Can you work these out from the model? Positions are in its coordinate system, mm. Give positions to 0.01 mm unless a question says otherwise; leave off trailing zeros. Loops run counter-clockwise (first coordinate to the right, second up) from the corner with the lowest first, then second, coordinate; pieces in that order, holes last. Notation, with made-up numbers: M 73,68 L 92,68 A11 ccw 92,81 Z; hole C 24.25,-26 d8. An arc over 180 degrees is marked long. Put each result on its own line as item: value. Start each with the question number.
1) For P1, Ø0.5, axis at y = 20.5, z = -0.5, coming from the -X side, with a flat end and sliding along its axis, tell me the tip position at first contact or that it passes through.
2) Imagine slicing it at B-B (x = 51.36). Write out the boundary of the cut face in (y, z), then the cut area to 3 significant figures.
3) Please list where these lines run through material, in increasing order: line 1 along X through (y, z) = (20.32, -0.7) (3 decimals); line 2 along X through (y, z) = (16.5, -0.75) (3 decimals); line 3 along Y through (x, z) = (48.5, -1.1). Write a range as from..to.
4) Imagine slicing it at C-C (z = -1.05). State how many separate pieces and enclosed holes the cut face has, then the cut area to 3 significant figures.
5) Imagine slicing it at A-A (y = 29.21). Write out the boundary of the cut face in (x, z) (3 decimals).
6) If we mould it in two halves opening along X, with no side actions, what happens to faces 1 (the cylindrical face through (17.4, 34.05, -0.79)), 2 (the cylindrical face through (52.055, 37.498, -0.789)), 3 (the cylindrical face through (45.35, 13.06, -0.79)), 4 (the flat face through (28, 19, -1.6))? For each: +X half, -X half, draft (parallel to the pull), parting line (faces both ways), or undercut.
from build123d import *

# Parameters (mm, degrees)
SKETCH_20_R         = 1.5
SKETCH_20_R_2       = 1.05
BOSS_EXTRUDE1_DEPTH = 1.6
SKETCH_17_R         = 0.8255
SKETCH_17_R_2       = 0.4191
SKETCH_17_R_3       = 0.41275
SKETCH_17_R_4       = 0.4699
SKETCH_17_R_5       = 0.829
CUT_EXTRUDE1_DEPTH  = 1.6


with BuildPart() as part:
    # Sketch 20 → Boss-Extrude1 (new body)
    with BuildSketch(Plane.XY):
        with BuildLine():
            Line((50.205, 38.4048), (6.31, 38.4048))
            ThreePointArc((6.31, 38.4048), (4.47911474, 37.520159965), (3.81, 35.6))
            Line((3.81, 35.6), (3.81, 2.5))
            ThreePointArc((3.81, 2.5), (4.542233047, 0.732233047), (6.31, 0))
            Line((6.31, 0), (50.205, 0))
            ThreePointArc((50.205, 0), (51.972766953, 0.732233047), (52.705, 2.5))
            Line((52.705, 2.5), (52.705, 35.6))
            ThreePointArc((52.705, 35.6), (52.03588526, 37.520159965), (50.205, 38.4048))
        make_face()
        with Locations((6.096, 2.1336)):
            Circle(SKETCH_20_R, mode=Mode.SUBTRACT)
        with Locations((50.5968, 2.1336)):
            Circle(SKETCH_20_R, mode=Mode.SUBTRACT)
        with Locations((50.5968, 36.2712)):
            Circle(SKETCH_20_R, mode=Mode.SUBTRACT)
        with Locations((6.096, 36.2712)):
            Circle(SKETCH_20_R, mode=Mode.SUBTRACT)
        with Locations((51.36, 12.26)):
            Circle(SKETCH_20_R_2, mode=Mode.SUBTRACT)
        with Locations((51.36, 20.76)):
            Circle(SKETCH_20_R_2, mode=Mode.SUBTRACT)
        with Locations((51.36, 24.96)):
            Circle(SKETCH_20_R_2, mode=Mode.SUBTRACT)
        with Locations((51.36, 33.46)):
            Circle(SKETCH_20_R_2, mode=Mode.SUBTRACT)
    extrude(amount=-BOSS_EXTRUDE1_DEPTH)

    # Sketch 17 → Cut-Extrude1 (cut)
    with BuildSketch(Plane.XY):
        with Locations((9.6012, 22.7838)):
            Circle(SKETCH_17_R)
        with Locations((12.319, 18.014)):
            Circle(SKETCH_17_R_2)
        with Locations((14.3002, 18.014)):
            Circle(SKETCH_17_R_2)
        with Locations((9.6012, 10.7442)):
            Circle(SKETCH_17_R)
        with Locations((20.066, 2.794)):
            Circle(SKETCH_17_R_3)
        with Locations((22.606, 2.794)):
            Circle(SKETCH_17_R_3)
        with Locations((25.146, 2.794)):
            Circle(SKETCH_17_R_3)
        with Locations((27.686, 2.794)):
            Circle(SKETCH_17_R_3)
        with Locations((22.606, 6.604)):
            Circle(SKETCH_17_R_3)
        with Locations((27.686, 6.604)):
            Circle(SKETCH_17_R_3)
        with Locations((17.145, 13.97)):
            Circle(SKETCH_17_R_3)
        with Locations((12.319, 15.514)):
            Circle(SKETCH_17_R_2)
        with Locations((14.3002, 15.514)):
            Circle(SKETCH_17_R_2)
        with Locations((14.605, 33.655)):
            Circle(SKETCH_17_R_4)
        with Locations((17.145, 33.655)):
            Circle(SKETCH_17_R_4)
        with Locations((19.685, 33.655)):
            Circle(SKETCH_17_R_4)
        with Locations((22.225, 33.655)):
            Circle(SKETCH_17_R_4)
        with Locations((24.765, 33.655)):
            Circle(SKETCH_17_R_4)
        with Locations((27.305, 33.655)):
            Circle(SKETCH_17_R_4)
        with Locations((29.845, 33.655)):
            Circle(SKETCH_17_R_4)
        with Locations((32.385, 33.655)):
            Circle(SKETCH_17_R_4)
        with Locations((34.925, 33.655)):
            Circle(SKETCH_17_R_4)
        with Locations((37.465, 33.655)):
            Circle(SKETCH_17_R_4)
        with Locations((40.005, 33.655)):
            Circle(SKETCH_17_R_4)
        with Locations((44.56, 32.91)):
            Circle(SKETCH_17_R_5)
        with Locations((48.26, 29.21)):
            Circle(SKETCH_17_R_5)
        with Locations((44.56, 25.51)):
            Circle(SKETCH_17_R_5)
        with Locations((44.56, 20.21)):
            Circle(SKETCH_17_R_5)
        with Locations((48.26, 16.51)):
            Circle(SKETCH_17_R_5)
        with Locations((44.56, 12.81)):
            Circle(SKETCH_17_R_5)
        with Locations((17.78, 20.32)):
            Circle(SKETCH_17_R_4)
        with Locations((17.78, 18.034)):
            Circle(SKETCH_17_R_4)
        with Locations((20.32, 20.32)):
            Circle(SKETCH_17_R_4)
        with Locations((20.32, 18.034)):
            Circle(SKETCH_17_R_4)
        with Locations((17.399, 11.049)):
            Circle(SKETCH_17_R_3)
        with Locations((19.685, 13.97)):
            Circle(SKETCH_17_R_3)
        with Locations((19.939, 11.049)):
            Circle(SKETCH_17_R_3)
        with Locations((22.86, 12.827)):
            Circle(SKETCH_17_R_4)
        with Locations((22.86, 10.287)):
            Circle(SKETCH_17_R_4)
    extrude(amount=-CUT_EXTRUDE1_DEPTH, mode=Mode.SUBTRACT)


solid = part.part
Recorded:
1. P1: x = 3.81
2. outline: M 0.28,-1.6 L 0.84,-1.6 L 0.84,0 L 0.28,0 Z; M 3.42,-1.6 L 11.21,-1.6 L 11.21,0 L 3.42,0 Z; M 13.31,-1.6 L 19.71,-1.6 L 19.71,0 L 13.31,0 Z; M 21.81,-1.6 L 23.91,-1.6 L 23.91,0 L 21.81,0 Z; M 26.01,-1.6 L 32.41,-1.6 L 32.41,0 L 26.01,0 Z; M 34.51,-1.6 L 34.98,-1.6 L 34.98,0 L 34.51,0 Z; M 37.56,-1.6 L 38.07,-1.6 L 38.07,0 L 37.56,0 Z
2. area: 38.7 mm²
3. line 1: 3.81..17.31, 18.25..19.85, 20.79..43.738, 45.382..50.407, 52.313..52.705
3. line 2: 3.81..47.431, 49.089..52.705
3. line 3: 0..15.72, 17.3..28.42, 30..38.4
4. separate pieces: 1
4. enclosed holes: 47
4. area: 1,790 mm²
5. outline: M 3.81,-1.6 L 47.431,-1.6 L 47.431,0 L 3.81,0 Z; M 49.089,-1.6 L 52.705,-1.6 L 52.705,0 L 49.089,0 Z
6. face 1: undercut
6. face 2: +X half
6. face 3: undercut
6. face 4: draft
